Build history of the part. All positions in model axes, mm. Face numbers are marked on the shaded views. A direction names the side the tool comes from. Coordinates: 2 decimals unless noted, no trailing zeros. Write each loop counter-clockwise with the first axis right and the second up, starting at its lowest first coordinate (ties: lowest second). Pieces come first, ordered by that corner, then holes.
```python
from build123d import *

# Parameters (mm, degrees)
F1_DEPTH = 3
F2_W     = 3
F2_H     = 25
F3_DEPTH = 25
F4_W     = 3
F4_H     = 25
F5_DEPTH = 25
F6_W     = 25
F6_H     = 15
F7_DEPTH = 3
F8_W     = 25
F8_H     = 15
F9_DEPTH = 3
F11_D    = 3.5
F13_D    = 8
F14_R    = 3
F15_R    = 6


with BuildPart() as f1:
    # F0 (on Top) → F1 (new body)
    with BuildSketch(Plane.XY):
        Polygon((-25, 0), (0, 0), (0, 51), (-25, 51), (-25, 45), (-51, 45), (-51, 6), (-25, 6), align=None)
    extrude(amount=F1_DEPTH)

    # F2 (on Right) → F3 (join)
    with BuildSketch(Plane.YZ):
        with Locations((1.5, -12.5)):
            Rectangle(F2_W, F2_H)
    extrude(amount=-F3_DEPTH)

    # F4 (on Right) → F5 (join)
    with BuildSketch(Plane.YZ):
        with Locations((49.5, -12.5)):
            Rectangle(F4_W, F4_H)
    extrude(amount=-F5_DEPTH)

    # F6 (on face) → F7 (join)
    with BuildSketch(Plane(origin=(0, 0, -25), x_dir=(1, 0, 0), z_dir=(0, 0, -1))):
        with Locations((-12.5, -7.5)):
            Rectangle(F6_W, F6_H)
    extrude(amount=-F7_DEPTH)

    # F8 (on face) → F9 (join)
    with BuildSketch(Plane(origin=(0, 0, -25), x_dir=(1, 0, 0), z_dir=(0, 0, -1))):
        with Locations((-12.5, -43.5)):
            Rectangle(F8_W, F8_H)
    extrude(amount=-F9_DEPTH)

    # F11 (through all)
    with Locations(Plane.XY.offset(3)):
        with Locations((-41, 41), (-10, 41), (-10, 10), (-41, 10)):
            Hole(F11_D / 2)

    # F13 (through all)
    with Locations(Plane.XY.offset(3)):
        with Locations((-25.5, 25.5)):
            Hole(F13_D / 2)

    # F14
    f14_edges = [f1.edges().sort_by_distance(p)[0] for p in [
        (-12.5, 3, 0),
        (-12.5, 48, 0),
        (-12.5, 48, -22),
        (-12.5, 3, -22),
    ]]
    fillet(f14_edges, radius=F14_R)

    # F15
    f15_edges = [f1.edges().sort_by_distance(p)[0] for p in [
        (-12.5, 0, 3),
        (-12.5, 0, -25),
        (-12.5, 51, 3),
        (-12.5, 51, -25),
    ]]
    fillet(f15_edges, radius=F15_R)


solid = f1.part
```
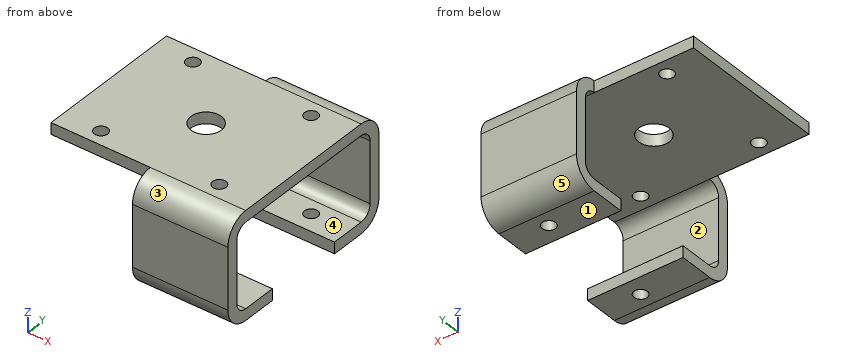
1. 3-axis set-ups, long thin cutter, end or side, ignore diameter. For the marked faces 1 and 2: which of +Z, -Z, +X, -X, +Y, -Y reach the whole face in a straight line?
Computed values:
face 1: -Z, +X, -X, +Y, -Y
face 2: +X, -X
2. Probe line 1 along Y through (x, z) = (-41, 2.2); line 2 along Y through (x, z) = (-21, -3.75); line 3 along Y through (x, z) = (-10, 1.95). List the from-to ranges inside material, lowest first.
Computed values:
line 1: y = 6 to 8.25, 11.75 to 39.25, 42.75 to 45
line 2: y = 0 to 3, 48 to 51
line 3: y = 2.61 to 8.25, 11.75 to 39.25, 42.75 to 48.39
3. Saw through at D-D on y = 10. List the corners of the cut face in (x, z), plus the area to 4 significant figures.
Computed values:
outline: (-51, 0) - (-42.75, 0) - (-42.75, 3) - (-51, 3) - close; (-39.25, 0) - (-11.75, 0) - (-11.75, 3) - (-39.25, 3) - close; (-25, -25) - (-11.75, -25) - (-11.75, -22) - (-25, -22) - close; (-8.25, -25) - (0, -25) - (0, -22) - (-8.25, -22) - close; (-8.25, 0) - (0, 0) - (0, 3) - (-8.25, 3) - close
area: 196.5 mm2
4. Mould opens along Y. For the marked faces 3, 4 and 5 say: +Y half, -Y half, draft (parallel to the pull), parting line (faces both ways), or undercut.
Computed values:
face 3: -Y half
face 4: undercut
face 5: +Y half
5. Saw through at A-A on y = 25.5. List the corners of the cut face in (x, z).
Computed values:
outline: (-51, 0) - (-29.5, 0) - (-29.5, 3) - (-51, 3) - close; (-21.5, 0) - (0, 0) - (0, 3) - (-21.5, 3) - close
6. Saw through at C-C on z = -8. List the corners of the cut face in (x, y).
Computed values:
outline: (-25, 0) - (0, 0) - (0, 3) - (-25, 3) - close; (-25, 48) - (0, 48) - (0, 51) - (-25, 51) - close
7. Flat gauge pins, fed straight in: pin 1 (12 mm diameter, centred on x = -34.5, y = 16.5, fed in from -Z); pin 2 (1.5 mm diameter, centred on x = -9, z = -23.5, fed in from -Y); pin 3 (7 mm diameter, centred on x = -11.5, y = 10, fed in from +Z); pin 4 (1.5 mm diameter, centred on x = -38, z = 1, fed in from -Y). Where does each tip first touch, or does it go through?
Computed values:
pin 1: stops at z = 0
pin 2: stops at y = 1.32
pin 3: stops at z = 3
pin 4: stops at y = 6
8. Saw through at B-B on x = -41. List the corners of the cut face in (y, z), plus the area to 3 significant figures.
Computed values:
outline: (6, 0) - (8.25, 0) - (8.25, 3) - (6, 3) - close; (11.75, 0) - (39.25, 0) - (39.25, 3) - (11.75, 3) - close; (42.75, 0) - (45, 0) - (45, 3) - (42.75, 3) - close
area: 96.0 mm2
